```python
from build123d import *

# Parameters (mm, degrees)
SKETCH1_W           = 3
SKETCH1_H           = 4
BOSS_EXTRUDE2_DEPTH = 3
FILLET1_R           = 8.464107


with BuildPart() as part:
    # Sketch1 → Boss-Extrude2 (new body)
    with BuildSketch(Plane(origin=(0, 0, 0), x_dir=(1, 0, 0), z_dir=(0, 1, 0))):
        with BuildLine():
            Line((-7.5, -42), (7.5, -42))
            Line((7.5, -42), (12.409150917, -1.504318289))
            ThreePointArc((12.409150917, -1.504318289), (0, 12.5), (-12.409150917, -1.504318289))
            Line((-12.409150917, -1.504318289), (-7.5, -42))
        make_face()
        with BuildLine():
            ThreePointArc((-1, -3.45), (-0.997357075, -3.377344208), (-0.989442272, -3.305072464))
            ThreePointArc((-0.989442272, -3.305072464), (0, 3.45), (0.989442272, -3.305072464))
            ThreePointArc((0.989442272, -3.305072464), (0.997357075, -3.377344208), (1, -3.45))
            Line((1, -3.45), (1, -13.45))
            ThreePointArc((1, -13.45), (0, -14.45), (-1, -13.45))
            Line((-1, -13.45), (-1, -3.45))
        make_face(mode=Mode.SUBTRACT)
        with Locations((-2.75, -35.1)):
            Rectangle(SKETCH1_W, SKETCH1_H, mode=Mode.SUBTRACT)
        with Locations((-2.75, -18.9)):
            Rectangle(SKETCH1_W, SKETCH1_H, mode=Mode.SUBTRACT)
        with Locations((2.75, -35.1)):
            Rectangle(SKETCH1_W, SKETCH1_H, mode=Mode.SUBTRACT)
        with Locations((2.75, -18.9)):
            Rectangle(SKETCH1_W, SKETCH1_H, mode=Mode.SUBTRACT)
    extrude(amount=BOSS_EXTRUDE2_DEPTH)

    # Fillet1
    fillet1_edges = [part.edges().sort_by_distance(p)[0] for p in [
        (-7.5, 1.5, 42),
        (7.5, 1.5, 42),
    ]]
    fillet(fillet1_edges, radius=FILLET1_R)


solid = part.part
```
Design review of the part built by this model. Coordinates are the model's own, in mm. A direction names the side the tool comes from. Coordinates: 2 decimals unless noted, no trailing zeros. Loops run counter-clockwise (first coordinate to the right, second up) from the corner with the lowest first, then second, coordinate; pieces in that order, holes last.
Q1. Tool access review of faces 4 (the face through (-5.549, 1.521, 39.927)), 5 (the face through (4.25, 1, 19)): name each direction out of +Z, -Z, +X, -X, +Y, -Y from which nothing blocks a thin tool from reaching the whole face with its end or side.
Reported:
face 4: +Z, -X, +Y, -Y
face 5: +Y, -Y
Q2. To check wall thickness, follow line 1 (X direction, y = 0.9, z = 0); line 2 (Z direction, x = -3, y = 1.85); line 3 (X direction, y = 2.6, z = 18.5). State the ranges of each line that lie inside material, in increasing order.
Reported:
line 1: x = -12.5 to -3.45, 3.45 to 12.5
line 2: z = -12.13 to -1.7, 1.7 to 16.9, 20.9 to 33.1, 37.1 to 41.45
line 3: x = -10.35 to -4.25, -1.25 to 1.25, 4.25 to 10.35
Q3. We need section C-C on x = 10.25. State the section outline as (y, z) points.
Reported:
outline: (0, -7.15) - (3, -7.15) - (3, 19.32) - (0, 19.32) - close
Q4. We need section A-A on y = 1.9. State how many separate pieces and enclosed holes the cut face has, and give its area (3 significant figures).
Reported:
separate pieces: 1
enclosed holes: 5
area: 959 mm2
Q5. The part is to be moulded in two halves that separate along Z. For faces 1 (the face through (-4.25, 1, 19)), 2 (the face through (-3, 3, 14)), 3 (the face through (5.549, 1.521, 39.927)), say which applies: +Z half, -Z half, draft (parallel to the pull), parting line (faces both ways), or undercut.
Reported:
face 1: undercut
face 2: draft
face 3: +Z half
Q6. We need section B-B on z = -7.5. State the section outline as (x, y) points.
Reported:
outline: (-10, 0) - (10, 0) - (10, 3) - (-10, 3) - close
Q7. For pin 1 (1.5 mm diameter, centred on y = 1.5, z = 18, fed in from -X); pin 2 (1.5 mm diameter, centred on y = 2, z = 19.5, fed in from +X), all flat-tipped, find the tip position at first contact; note any pin that passes through.
Reported:
pin 1: stops at x = -10.5
pin 2: stops at x = 10.32
